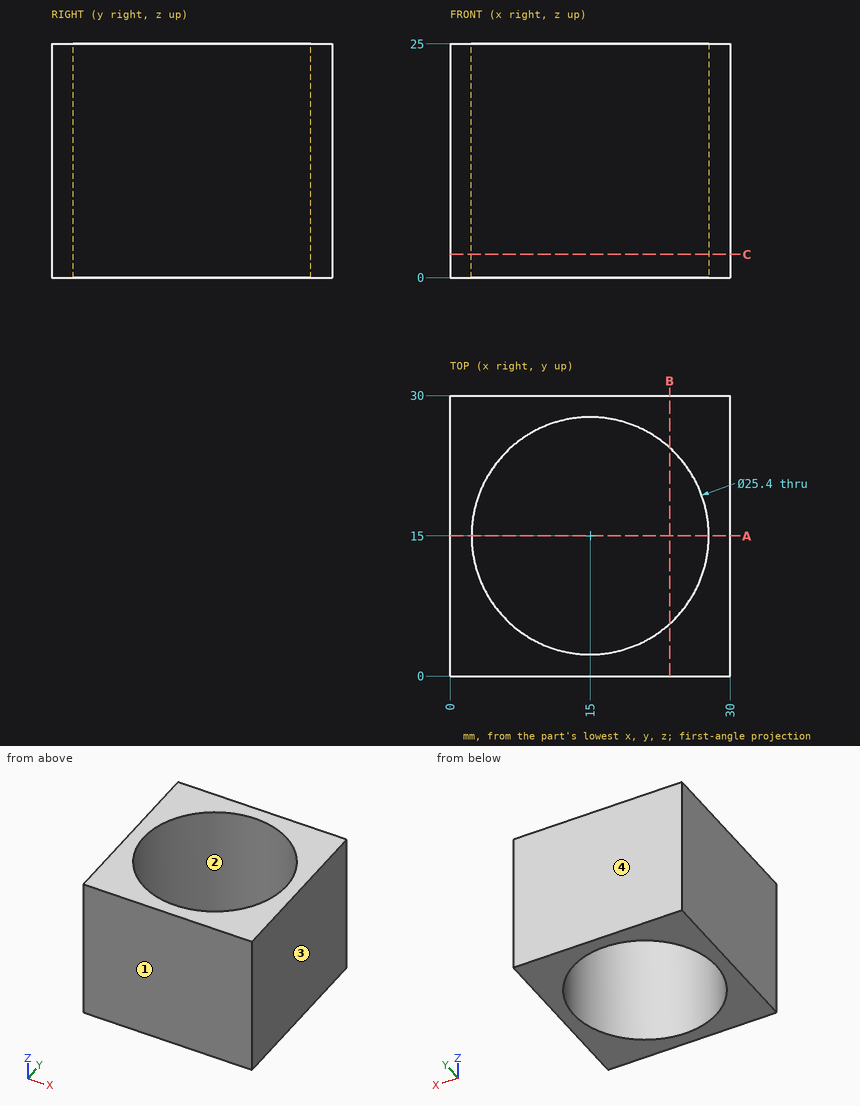
Check sheet for the drawn part. Datum: minimum x, y, z corner. Units: mm. Round coordinates to 2 decimals unless told otherwise and drop trailing zeros. Loops run counter-clockwise (first coordinate to the right, second up) from the corner with the lowest first, then second, coordinate; pieces in that order, holes last. Notation, with made-up numbers: (5, -38.5) - (46, -38.5) arc R15 ccw to (46, -23.5) - close; hole circle Ø7 at (61, -15.5). An arc over 180 degrees is marked (long way). Answer as a JSON object with one key per item and string values. Group by question number.
Q1. Sectioned sample at B-B, the plane x = 23.5. Enter the section's corners in (y, z).
Q2. Gauge pin test, flat end, axial feed: P1, Ø1.5, axis at x = 6.5, y = 21.5, coming from the +Z side. Record the tip position at first contact, or that the pin passes through.
Q3. Sectioned sample at A-A, the plane y = 15. Enter the section's corners in (x, z).
Q4. Scan lines: line 1 along Y through (x, z) = (15, 14.25); line 2 along Y through (x, z) = (23.75, 6.25); line 3 along X through (y, z) = (9.5, 12.25). Record each from-to range of solid material in increasing order. Write a range as [from, to].
Q5. Sectioned sample at C-C, the plane z = 2.5. Enter the section's corners in (x, y), plus the area to 3 significant figures.
Q6. Mould release check, pull along Y, two halves, no side actions. Record for the marked faces 1, 2, 3 and 4: released by +Y, released by -Y, zero draft, split by the parting line, or undercut.
Solution:
{
 "1": {"outline": "(0, 0) - (5.56, 0) - (5.56, 25) - (0, 25) - close; (24.44, 0) - (30, 0) - (30, 25) - (24.44, 25) - close"},
 "2": {"P1": "passes through"},
 "3": {"outline": "(0, 0) - (2.3, 0) - (2.3, 25) - (0, 25) - close; (27.7, 0) - (30, 0) - (30, 25) - (27.7, 25) - close"},
 "4": {"line 1": "y = [0, 2.3], [27.7, 30]", "line 2": "y = [0, 5.8], [24.2, 30]", "line 3": "x = [0, 3.55], [26.45, 30]"},
 "5": {"outline": "(0, 0) - (30, 0) - (30, 30) - (0, 30) - close; hole circle Ø25.4 at (15, 15)", "area": "393 mm²"},
 "6": {"face 1": "released by -Y", "face 2": "undercut", "face 3": "zero draft", "face 4": "released by +Y"}
}
